```python
from build123d import *

# Parameters (mm, degrees)
CROQUIS1_R              = 0.75
CROQUIS1_R_2            = 0.5
SALIENTE_EXTRUIR1_DEPTH = 0.2


with BuildPart() as part:
    # Croquis1 → Saliente-Extruir1 (new body)
    with BuildSketch(Plane.XY):
        with BuildLine():
            Line((0.480813239, 0.57560284), (0, 15))
            Line((0, 15), (-0.480813239, 0.57560284))
            ThreePointArc((-0.480813239, 0.57560284), (0, 0.75), (0.480813239, 0.57560284))
        make_face()
        Circle(CROQUIS1_R)
        Circle(CROQUIS1_R_2, mode=Mode.SUBTRACT)
        with BuildLine():
            ThreePointArc((0.518076883, -0.542306503), (0, -0.75), (-0.518076883, -0.542306503))
            Line((-0.518076883, -0.542306503), (-0.6, -3))
            add(Edge.make_bspline(
                [(-0.6, -3), (-0.201744862, -2.954169047), (0.201744862, -2.954169047), (0.6, -3)],
                knots=[0.345361209, 0.345361209, 0.345361209, 0.345361209, 0.654638791, 0.654638791, 0.654638791, 0.654638791], degree=3))
            Line((0.6, -3), (0.518076883, -0.542306503))
        make_face()
        with BuildLine():
            add(Edge.make_bspline(
                [(-0.6, -3), (-0.201744862, -2.954169047), (0.201744862, -2.954169047), (0.6, -3)],
                knots=[0.345361209, 0.345361209, 0.345361209, 0.345361209, 0.654638791, 0.654638791, 0.654638791, 0.654638791], degree=3))
            add(Edge.make_bspline(
                [(-1.9, -3.324981437), (-1.482912392, -3.159505228), (-1.044719839, -3.051178082), (-0.6, -3)],
                knots=[0, 0, 0, 0, 0.345361209, 0.345361209, 0.345361209, 0.345361209], degree=3))
            Line((-1.9, -3.324981437), (-1.71561069, -3.789740065))
            add(Edge.make_bspline(
                [(-1.71561069, -3.789740065), (-0.652484196, -3.367953038), (0.652484196, -3.367953038), (1.71561069, -3.789740065)],
                knots=[0, 0, 0, 0, 1, 1, 1, 1], degree=3))
            Line((1.71561069, -3.789740065), (1.9, -3.324981437))
            add(Edge.make_bspline(
                [(0.6, -3), (1.044719839, -3.051178082), (1.482912392, -3.159505228), (1.9, -3.324981437)],
                knots=[0.654638791, 0.654638791, 0.654638791, 0.654638791, 1, 1, 1, 1], degree=3))
        make_face()
    extrude(amount=SALIENTE_EXTRUIR1_DEPTH)


solid = part.part
```
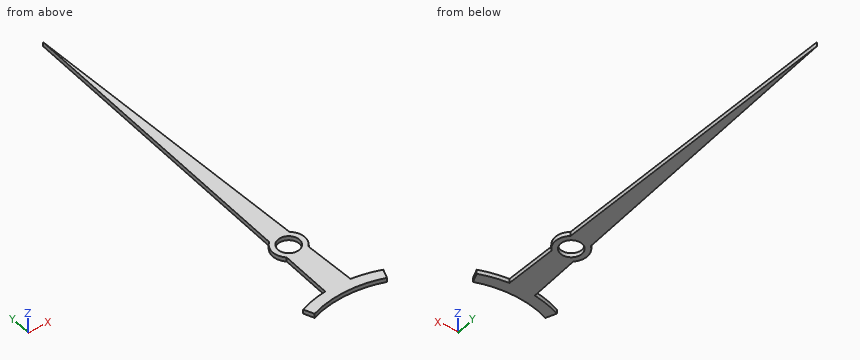
Check sheet for the modelled part. Datum: model origin and axes. Units: mm. Round coordinates to 2 decimals unless told otherwise and drop trailing zeros. Order: outer loops, then holes, each group sorted by start corner. A loop starts at its lowest first (then second) coordinate and runs counter-clockwise, first axis right, second up.
1) Scan lines: line 1 (Y direction, x = -0.95, z = 0.1); line 2 (Y direction, x = 1.45, z = 0.15); line 3 (X direction, y = 11, z = 0.15). Record each from-to range of solid material in increasing order.
2) Section check C-C (y = -2). Record the boundary of the cut face in (x, z).
3) Section check A-A (y = 0). Record the boundary of the cut face in (x, z), and give its area (3 significant figures).
4) Go/stop test with a flat-tipped pin: pin 1 Ø1 at (x, y) = (1, 10.5) entering from -Z. Record where the tip stops, or that it passes through.
5) Section check B-B (y = 13.5). Record the boundary of the cut face in (x, z), and give its area (3 significant figures).
Result:
1. line 1: y = -3.57 to -3.05
1. line 2: y = -3.69 to -3.17
1. line 3: x = -0.13 to 0.13
2. outline: (-0.57, 0) - (0.57, 0) - (0.57, 0.2) - (-0.57, 0.2) - close
3. outline: (-0.75, 0) - (-0.5, 0) - (-0.5, 0.2) - (-0.75, 0.2) - close; (0.5, 0) - (0.75, 0) - (0.75, 0.2) - (0.5, 0.2) - close
3. area: 0.100 mm2
4. pin 1: passes through
5. outline: (-0.05, 0) - (0.05, 0) - (0.05, 0.2) - (-0.05, 0.2) - close
5. area: 0.0200 mm2
